Design review of the part built by this model. Coordinates are the model's own, in mm. Give positions to 0.01 mm unless a question says otherwise; leave off trailing zeros. Loops run counter-clockwise (first coordinate to the right, second up) from the corner with the lowest first, then second, coordinate; pieces in that order, holes last. Notation, with made-up numbers: (-7, 39) -> (41, 39) arc R23 cw to (41, 65) -> close; hole circle Ø6 at (-2.5, 74). An arc over 180 degrees is marked (long way). Use a Markdown table: item, result. Add a question column.
1. Add section A-A (x = -19.05). State the section outline as (y, z) points (3 decimals), and give its area (3 significant figures).
2. For pin 1 Ø1.6 at (y, z) = (35, 1.5) entering from +X; pin 2 Ø5.5 at (x, y) = (19.05, -38.1) entering from -Z; pin 3 Ø1 at (x, z) = (23, 1) entering from -Y; pin 4 Ø1.5 at (y, z) = (-35, 2) entering from +X, all flat-tipped, find the tip position at first contact; note any pin that passes through.
3. Add section C-C (y = 52). State the section outline as (x, z) points (3 decimals), and give its area (3 significant figures).
4. Add section B-B (z = 0.85). State the section outline as (x, y) points.
5. To check wall thickness, follow line 1 (X direction, y = 38.1, z = 1.3); line 2 (X direction, y = -31.75, z = 1.5); line 3 (Y direction, x = -19.05, z = 1.75). State the ranges of each line that lie inside material, in increasing order.
6. Add section D-D (x = 34). State the section outline as (y, z) points (3 decimals).
Autodesk Inventor part; units mm, degrees
ref_plane "YZ Plane" through (0, 0, 0) normal (1, 0, 0) x (0, 1, 0)
ref_plane "XZ Plane" through (0, 0, 0) normal (0, 1, 0) x (-1, 0, 0)
ref_plane "XY Plane" through (0, 0, 0) normal (0, 0, 1) x (1, 0, 0)
sketch "Sketch1" plane through (0, 0, 0) normal (0, 0, 1) x (1, 0, 0)
  line L0 (19.05, 38.1) -> (-19.05, 38.1) construction
  line L1 (-19.05, 38.1) -> (-19.05, -38.1) construction
  line L2 (-19.05, -38.1) -> (19.05, -38.1) construction
  line L3 (19.05, -38.1) -> (19.05, 38.1) construction
  line L4 (19.05, 38.1) -> (-19.05, -38.1) construction
  line L5 (-19.05, 38.1) -> (19.05, -38.1) construction
  line L6 (-50.8, -69.85) -> (38.1, -69.85)
  line L7 (50.8, -57.15) -> (50.8, 57.15)
  line L8 (38.1, 69.85) -> (-38.1, 69.85)
  line L9 (-50.8, 57.15) -> (-50.8, -69.85)
  line L10 (-50.8, -69.85) -> (50.8, 69.85) construction
  line L11 (50.8, -69.85) -> (-50.8, 69.85) construction
  circle A0 centre (18.4474, 77.2895) radius 12.7
  circle A1 centre (63.5, -31.75) radius 12.7
  circle A2 centre (-38.1, -107.95) radius 12.7
  arc A3 (-6.4019, 69.85) -> (6.0228, 79.9198) centre (-6.4019, 82.55) ccw
  arc A4 (50.8, -6.35) -> (63.5, -19.05) centre (63.5, -6.35) ccw
  arc A5 (63.5, -44.45) -> (50.8, -57.15) centre (63.5, -57.15) ccw
  arc A6 (12.7, -69.85) -> (-25.4, -107.95) centre (12.7, -107.95) ccw
  line L12 (-50.8, -107.95) -> (-50.8, -69.85)
  arc A7 (38.1, -69.85) -> (50.8, -57.15) centre (38.1, -57.15) ccw
  arc A8 (50.8, 57.15) -> (38.1, 69.85) centre (38.1, 57.15) ccw
  arc A9 (-38.1, 69.85) -> (-50.8, 57.15) centre (-38.1, 57.15) ccw
  arc A10 (19.9641, 75.8806) -> (17.0385, 78.8062) centre (18.4474, 77.2895) ccw
  arc A11 (50.8, 57.15) -> (18.7582, 89.9857) centre (17.9544, 57.15) ccw
  point P0 (0, 0)
  point P1 (-38.1, -69.85)
  point P2 (-50.8, -78.4346)
  point P3 (50.8, -31.75)
  point P4 (8.1546, 69.85)
  point P5 (28.7403, 69.85)
  dimension "d0" = 38.1
  dimension "d1" = 76.2
  dimension "d2" = 31.75
  dimension "d3" = 31.75
  dimension "d13" = 25.4
  dimension "d20" = 12.7
  dimension "d21" = 76.2
  dimension "d22" = 38.1
  dimension "d23" = 32.8456
extrude "Extrusion1" add sketch "Sketch1" along normal blind 3.175
hole "Hole1" at (-19.05, 38.1, 0) at (19.05, 38.1, 0) at (19.05, -38.1, 0) at (-19.05, -38.1, 0) at (-38.1, -107.95, 0) at (63.5, -31.75, 0) at (18.4474, 77.2895, 0) direction (0, 0, 1) diameter 4.572 end through all
properties part number "Brain Mount"
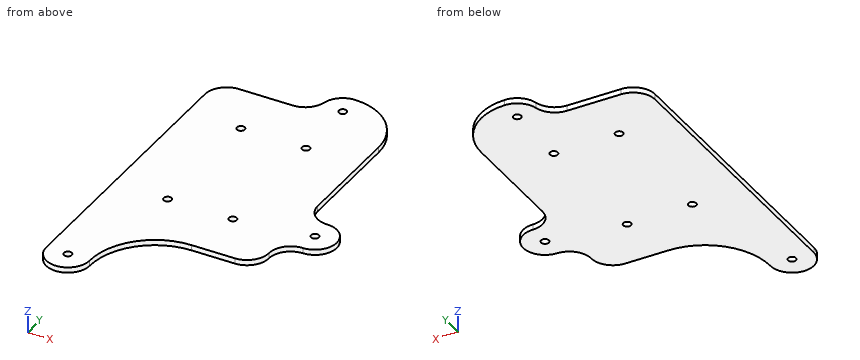
Taken from the geometry:
| question | item | result |
|---|---|---|
| 1 | outline | (-86.889, 0) -> (-40.386, 0) -> (-40.386, 3.175) -> (-86.889, 3.175) -> close; (-35.814, 0) -> (35.814, 0) -> (35.814, 3.175) -> (-35.814, 3.175) -> close; (40.386, 0) -> (69.85, 0) -> (69.85, 3.175) -> (40.386, 3.175) -> close |
| 1 | area | 469 mm^2 |
| 2 | pin 1 | stops at x = 50.8 |
| 2 | pin 2 | stops at z = 0 |
| 2 | pin 3 | stops at y = -69.85 |
| 2 | pin 4 | stops at x = 75.95 |
| 3 | outline | (-50.8, 0) -> (50.8, 0) -> (50.8, 3.175) -> (-50.8, 3.175) -> close |
| 3 | area | 323 mm^2 |
| 4 | outline | (-50.8, -107.95) arc R12.7 ccw to (-25.4, -107.95) arc R38.1 cw to (12.7, -69.85) -> (38.1, -69.85) arc R12.7 ccw to (50.8, -57.15) arc R12.7 cw to (63.5, -44.45) arc R12.7 ccw to (63.5, -19.05) arc R12.7 cw to (50.8, -6.35) -> (50.8, 57.15) arc R32.85 ccw to (18.76, 89.99) arc R12.7 ccw to (6.02, 79.92) arc R12.7 cw to (-6.4, 69.85) -> (-38.1, 69.85) arc R12.7 ccw to (-50.8, 57.15) -> close; hole circle Ø4.57 at (-38.1, -107.95); hole circle Ø4.57 at (-19.05, -38.1); hole circle Ø4.57 at (-19.05, 38.1); hole circle Ø4.57 at (18.45, 77.29); hole circle Ø4.57 at (19.05, -38.1); hole circle Ø4.57 at (19.05, 38.1); hole circle Ø4.57 at (63.5, -31.75) |
| 5 | line 1 | x = -50.8 to -21.34, -16.76 to 16.76, 21.34 to 50.8 |
| 5 | line 2 | x = -50.8 to 61.21, 65.79 to 76.2 |
| 5 | line 3 | y = -86.89 to -40.39, -35.81 to 35.81, 40.39 to 69.85 |
| 6 | outline | (-69.85, 0) -> (85.81, 0) -> (85.81, 3.175) -> (-69.85, 3.175) -> close |
